Geometry: see drawing. Coordinates: mm, zero at the bounding-box minimum. A direction names the side the tool comes from. Coordinates: 2 decimals unless noted, no trailing zeros. Loops run counter-clockwise (first coordinate to the right, second up) from the corner with the lowest first, then second, coordinate; pieces in that order, holes last. Notation, with made-up numbers: (89, -16.5) - (114, -16.5) arc R26 ccw to (114, 10.5) - close; hole circle Ø2 at (57, -19.75). An arc over 180 degrees is marked (long way). Answer in a Markdown table with one row per item.
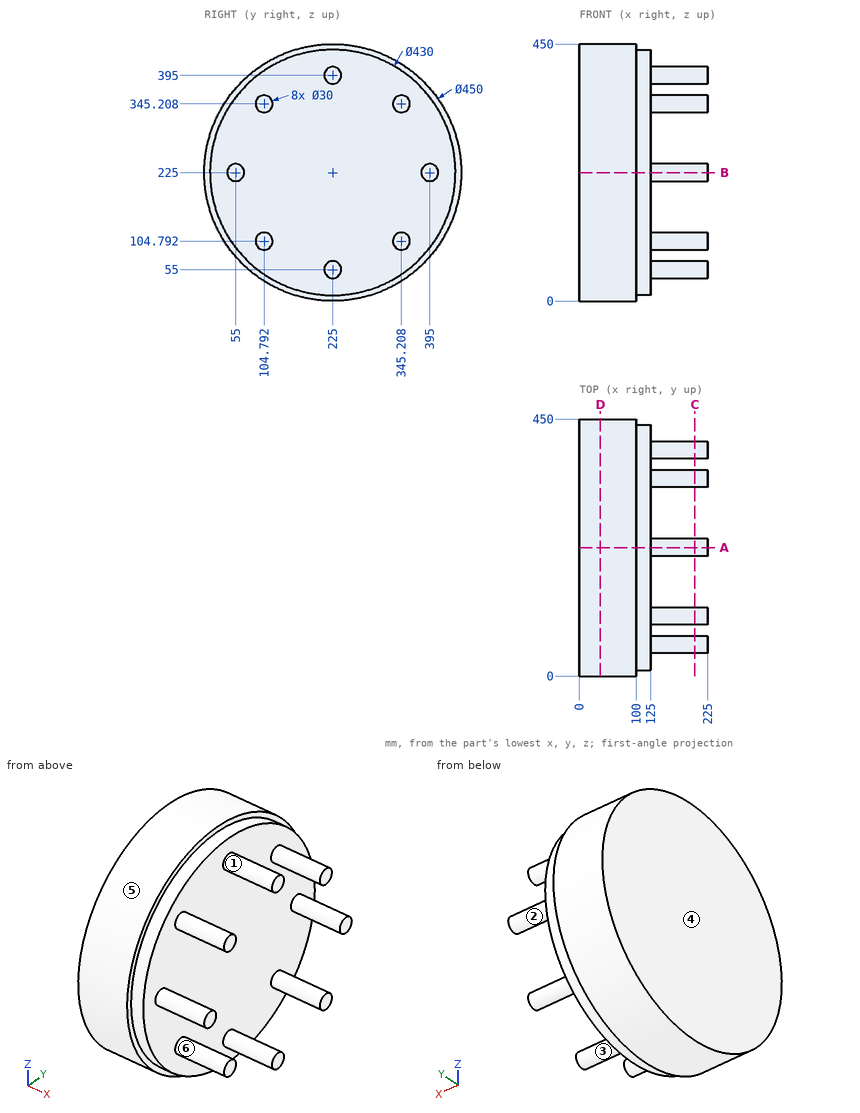
(1) Ray query, probe 1 along X at (y, z) = (127, 143); probe 2 along Z at (x, y) = (179, 223); probe 3 along Z at (x, y) = (109.5, 218). Return the intervals inside material, ascending.
Verdict:
| item | result |
|---|---|
| probe 1 | x = 0 to 125 |
| probe 2 | z = 40.13 to 69.87, 380.13 to 409.87 |
| probe 3 | z = 10.11 to 439.89 |
(2) Cut plane A-A on y = 225. Output: boundary loops of the cut face in (x, z), then the cut area to 4 significant figures.
Verdict:
| item | result |
|---|---|
| outline | (0, 0) - (100, 0) - (100, 10) - (125, 10) - (125, 40) - (225, 40) - (225, 70) - (125, 70) - (125, 380) - (225, 380) - (225, 410) - (125, 410) - (125, 440) - (100, 440) - (100, 450) - (0, 450) - close |
| area | 61,750 mm² |
(3) Access query for the marked faces 5 and 6. Directions: +Z, -Z, +X, -X, +Y, -Y. A direction counts if a zero-diameter tool reaches every point of the face in a straight line with its end or side. Return the directions, or none.
Verdict:
| item | result |
|---|---|
| face 5 | +X, -X |
| face 6 | +X |
(4) Pull-direction query (Z, two-part tool) for the marked faces 1, 2, 3 and 4; classes: pulls with the +Z half, pulls with the -Z half, needs draft (parallel to the pull), parting line crosses it, or undercut.
Verdict:
| item | result |
|---|---|
| face 1 | undercut |
| face 2 | parting line crosses it |
| face 3 | undercut |
| face 4 | needs draft |
(5) Cut plane D-D on x = 37. Output: boundary loops of the cut face in (y, z), then the cut area to 3 significant figures.
Verdict:
| item | result |
|---|---|
| outline | circle Ø450 at (225, 225) |
| area | 159,000 mm² |
(6) First-contact query: pin 1 Ø10 at (x, z) = (190, 343.5) entering from -Y; pin 2 Ø5 at (x, z) = (56.5, 108) entering from +Y; pin 3 Ø8 at (y, z) = (358.5, 189.5) entering from +X. Flat tips, straight axial feed; report the tip coordinate or a pass-through.
Verdict:
| item | result |
|---|---|
| pin 1 | stops at y = 89.79 |
| pin 2 | stops at y = 418.69 |
| pin 3 | stops at x = 125 |
(7) Cut plane C-C on x = 202.5. Output: boundary loops of the cut face in (y, z), then the cut area to 4 significant figures.
Verdict:
| item | result |
|---|---|
| outline | circle Ø30 at (55, 225); circle Ø30 at (104.79, 104.79); circle Ø30 at (104.79, 345.21); circle Ø30 at (225, 55); circle Ø30 at (225, 395); circle Ø30 at (345.21, 104.79); circle Ø30 at (345.21, 345.21); circle Ø30 at (395, 225) |
| area | 5,655 mm² |
